Could you check a few things on this model? Use its own coordinates, in mm. Face numbers are marked on the shaded views. A direction names the side the tool comes from. Give positions to 0.01 mm unless a question says otherwise; leave off trailing zeros. Write each loop counter-clockwise with the first axis right and the second up, starting at its lowest first coordinate (ties: lowest second). Pieces come first, ordered by that corner, then holes. Notation, with made-up numbers: (-4, 61.25) - (54, 61.25) arc R32 cw to (54, 88.25) - close; hole circle Ø8 at (-27, 64). An arc over 180 degrees is marked (long way). Answer as CSV lines item,"result". Start each with the question number.
Q1. If I drill on line 1 along X through (y, z) = (6.4, -10.56); line 2 along X through (y, z) = (2.1, -10.56); line 3 along Z through (x, y) = (28.01, 1.75), over which ranges is the centre line in solid material (lowest first)?
Q2. Will these pins go through, and if not, where does the flat tip stop? pin 1 Ø1.6 at (y, z) = (9, -6) entering from -X; pin 2 Ø5.5 at (x, z) = (28.01, -10.56) entering from +Y; pin 3 Ø4 at (x, z) = (12, -6) entering from +Y.
Q3. Imagine slicing it at A-A on y = 4. List the corners of the cut face in (x, z) for me.
Q4. On a 3-axis mill with a long thin cutter (end or side, diameter ignored), from which of +Z, -Z, +X, -X, +Y, -Y can I reach the whole of each face in a straight line? I mean the marked faces 1 and 2. Say none if no direction works.
Q5. Imagine slicing it at D-D on x = 5. List the corners of the cut face in (y, z) for me.
Q6. We'd pull the mould along Z, two halves only. Please class the marked faces 3, 4, 5 and 6: pulls with the +Z half, pulls with the -Z half, needs draft (parallel to the pull), parting line crosses it, or undercut.
Q7. Imagine slicing it at B-B on z = -15.5. List the corners of the cut face in (x, y) for me, and give its area (3 significant figures).
Q8. Imagine slicing it at C-C on x = 28.01. List the corners of the cut face in (y, z) for me.
```python
from build123d import *

# Parameters (mm, degrees)
SKETCH1_W           = 39
SKETCH1_H           = 21
BOSS_EXTRUDE1_DEPTH = 7.5
SKETCH2_W           = 37
SKETCH2_H           = 19
CUT_EXTRUDE1_DEPTH  = 6.5
FILLET1_R           = 1
FILLET2_R           = 1
SKETCH3_W           = 37
SKETCH3_H           = 19
BOSS_EXTRUDE2_DEPTH = 8.5
SKETCH4_W           = 35
SKETCH4_H           = 17
CUT_EXTRUDE2_DEPTH  = 8.5
SKETCH5_R           = 4
BOSS_EXTRUDE3_DEPTH = 6.5
SKETCH6_R           = 3
CUT_EXTRUDE3_DEPTH  = 7.5
SKETCH7_R           = 4
BOSS_EXTRUDE4_DEPTH = 4
SKETCH8_R           = 1.75
CUT_EXTRUDE4_DEPTH  = 4
CUT_EXTRUDE5_DEPTH  = 2


with BuildPart() as part:
    # Sketch1 → Boss-Extrude1 (new body)
    with BuildSketch(Plane(origin=(0, 0, 0), x_dir=(1, 0, 0), z_dir=(0, 1, 0))):
        with Locations((19.5, 10.5)):
            Rectangle(SKETCH1_W, SKETCH1_H)
    extrude(amount=BOSS_EXTRUDE1_DEPTH)

    # Sketch2 → Cut-Extrude1 (cut)
    with BuildSketch(Plane(origin=(0, 7.5, 0), x_dir=(1, 0, 0), z_dir=(0, 1, 0))):
        with Locations((19.5, 10.5)):
            Rectangle(SKETCH2_W, SKETCH2_H)
    extrude(amount=-CUT_EXTRUDE1_DEPTH, mode=Mode.SUBTRACT)

    # Fillet1
    fillet1_edges = [part.edges().sort_by_distance(p)[0] for p in [
        (0, 3.75, -21),
        (39, 3.75, -21),
        (39, 3.75, 0),
        (0, 3.75, 0),
    ]]
    fillet(fillet1_edges, radius=FILLET1_R)

    # Fillet2
    fillet2_edges = [part.edges().sort_by_distance(p)[0] for p in [
        (39, 0, -10.5),
        (0, 0, -10.5),
        (19.5, 0, -21),
        (19.5, 0, 0),
        (0.292893219, 0, -0.292893219),
        (0.292893219, 0, -20.707106781),
        (38.707106781, 0, -20.707106781),
        (38.707106781, 0, -0.292893219),
    ]]
    fillet(fillet2_edges, radius=FILLET2_R)

    # Sketch3 → Boss-Extrude2 (add)
    with BuildSketch(Plane(origin=(0, 1, 0), x_dir=(1, 0, 0), z_dir=(0, 1, 0))):
        with Locations((19.5, 10.5)):
            Rectangle(SKETCH3_W, SKETCH3_H)
    extrude(amount=BOSS_EXTRUDE2_DEPTH)

    # Sketch4 → Cut-Extrude2 (cut)
    with BuildSketch(Plane(origin=(0, 9.5, 0), x_dir=(1, 0, 0), z_dir=(0, 1, 0))):
        with Locations((19.5, 10.5)):
            Rectangle(SKETCH4_W, SKETCH4_H)
    extrude(amount=-CUT_EXTRUDE2_DEPTH, mode=Mode.SUBTRACT)

    # Sketch5 → Boss-Extrude3 (add)
    with BuildSketch(Plane(origin=(0, 1, 0), x_dir=(1, 0, 0), z_dir=(0, 1, 0))):
        with Locations((28.01, 10.56)):
            Circle(SKETCH5_R)
    extrude(amount=BOSS_EXTRUDE3_DEPTH)

    # Sketch6 → Cut-Extrude3 (cut)
    with BuildSketch(Plane(origin=(0, 7.5, 0), x_dir=(1, 0, 0), z_dir=(0, 1, 0))):
        with Locations((28.01, 10.56)):
            Circle(SKETCH6_R)
    extrude(amount=-CUT_EXTRUDE3_DEPTH, mode=Mode.SUBTRACT)

    # Sketch7 → Boss-Extrude4 (add)
    with BuildSketch(Plane(origin=(0, 7.5, 0), x_dir=(1, 0, 0), z_dir=(0, 1, 0))):
        with Locations((28.01, 10.56)):
            Circle(SKETCH7_R)
    extrude(amount=-BOSS_EXTRUDE4_DEPTH)

    # Sketch8 → Cut-Extrude4 (cut)
    with BuildSketch(Plane(origin=(0, 7.5, 0), x_dir=(1, 0, 0), z_dir=(0, 1, 0))):
        with Locations((28.01, 10.56)):
            Circle(SKETCH8_R)
    extrude(amount=-CUT_EXTRUDE4_DEPTH, mode=Mode.SUBTRACT)

    # Sketch9 → Cut-Extrude5 (cut)
    with BuildSketch(Plane(origin=(39, 0, 0), x_dir=(0, 0, -1), z_dir=(1, 0, 0))):
        with BuildLine():
            Line((8.5, 7.5), (8.5, 9.5))
            Line((8.5, 9.5), (12.5, 9.5))
            Line((12.5, 9.5), (12.5, 7.5))
            ThreePointArc((12.5, 7.5), (10.5, 5.5), (8.5, 7.5))
        make_face()
    extrude(amount=-CUT_EXTRUDE5_DEPTH, mode=Mode.SUBTRACT)


solid = part.part
```
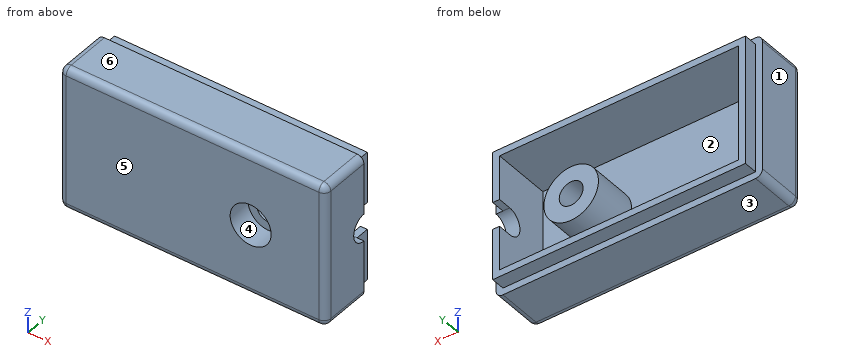
Conclusion:
1,line 1,"0 to 2, 24.01 to 26.26, 29.76 to 32.01"
1,line 2,"0 to 2, 24.01 to 25.01, 31.01 to 32.01, 37 to 39"
1,line 3,"-21 to -19, -14.56 to -13.56, -7.56 to -6.56, -2 to 0"
2,pin 1,"x = 1"
2,pin 2,"y = 7.5"
2,pin 3,"y = 1"
3,outline,"(0, -20) arc R1 ccw to (1, -21) - (38, -21) arc R1 ccw to (39, -20) - (39, -1) arc R1 ccw to (38, 0) - (1, 0) arc R1 ccw to (0, -1) - close; circle Ø8 at (28.01, -10.56); hole (2, -19) - (37, -19) - (37, -2) - (2, -2) - close; hole circle Ø3.5 at (28.01, -10.56)"
4,face 1,"+Z, -Z, -X, +Y, -Y"
4,face 2,"+Y"
5,outline,"(0, -20) arc R1 ccw to (1, -21) - (7.5, -21) - (7.5, -20) - (9.5, -20) - (9.5, -19) - (1, -19) - (1, -2) - (9.5, -2) - (9.5, -1) - (7.5, -1) - (7.5, 0) - (1, 0) arc R1 ccw to (0, -1) - close"
6,face 3,"pulls with the -Z half"
6,face 4,"undercut"
6,face 5,"needs draft"
6,face 6,"pulls with the +Z half"
7,outline,"(0, 1) arc R1 ccw to (1, 0) - (38, 0) arc R1 ccw to (39, 1) - (39, 7.5) - (38, 7.5) - (38, 9.5) - (37, 9.5) - (37, 1) - (2, 1) - (2, 9.5) - (1, 9.5) - (1, 7.5) - (0, 7.5) - close"
7,area,"68.6 mm^2"
8,outline,"(0, -20) arc R1 ccw to (1, -21) - (7.5, -21) - (7.5, -20) - (9.5, -20) - (9.5, -19) - (1, -19) - (1, -14.56) - (7.5, -14.56) - (7.5, -12.31) - (3.5, -12.31) - (3.5, -13.56) - (0, -13.56) - close; (0, -7.56) - (3.5, -7.56) - (3.5, -8.81) - (7.5, -8.81) - (7.5, -6.56) - (1, -6.56) - (1, -2) - (9.5, -2) - (9.5, -1) - (7.5, -1) - (7.5, 0) - (1, 0) arc R1 ccw to (0, -1) - close"
